For this review, use the dimensioned drawing (mm, ordinates from the lowest corner) and the shaded views. A direction names the side the tool comes from. Coordinates: 2 decimals unless noted, no trailing zeros. Order: outer loops, then holes, each group sorted by start corner. A loop starts at its lowest first (then second) coordinate and runs counter-clockwise, first axis right, second up. Notation, with made-up numbers: M 34.25,47 L 62.25,47 A19 cw 62.25,54 Z; hole C 22,34 d5. An arc over 180 degrees is marked long. Answer in a Markdown table with one row per item.
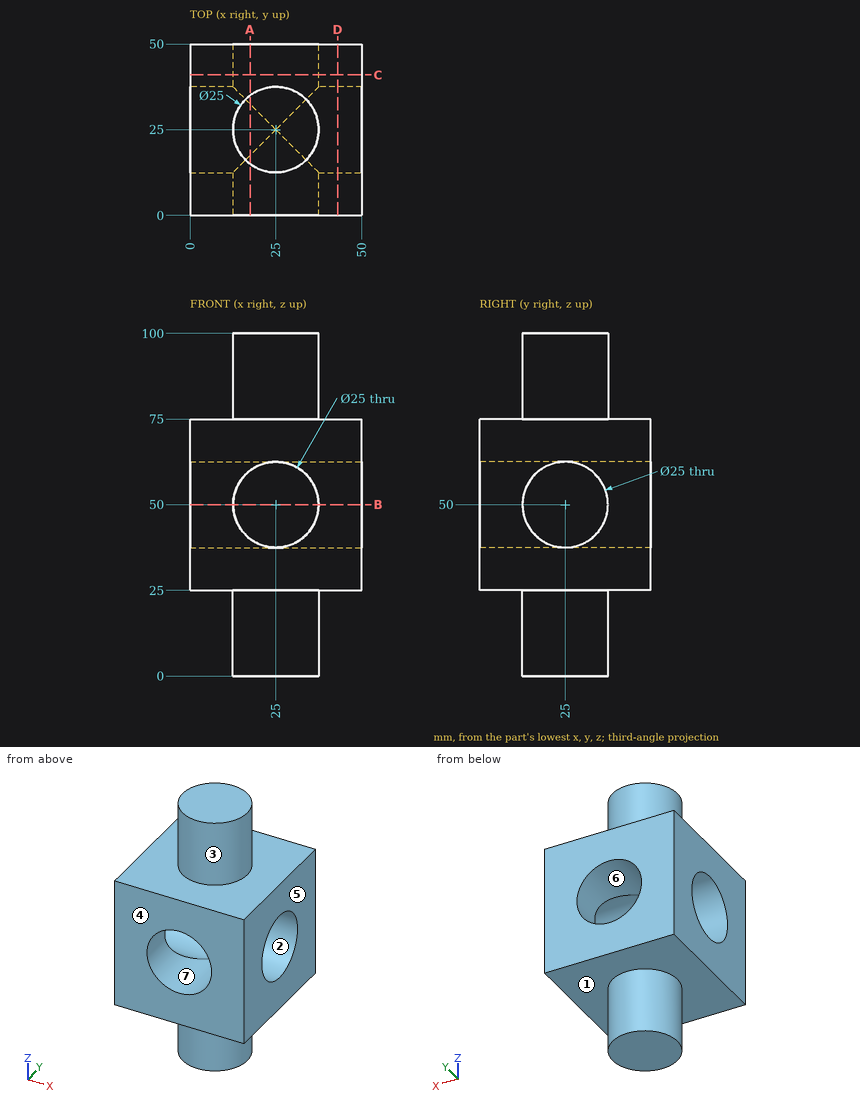
(1) Take a section at C-C (y = 41). Write out the cut boundary in (x, z), then the cut area to 3 significant figures.
Report:
| item | result |
|---|---|
| outline | M 0,25 L 50,25 L 50,75 L 0,75 Z; hole C 25,50 d25 |
| area | 2,010 mm^2 |
(2) Insertion check: P1, Ø8, axis at x = 10.5, y = 16, coming from the +Z side; P2, Ø15, axis at x = 25, z = 50, coming from the +Y side; P3, Ø6, axis at x = 35.5, z = 60.5, coming from the -Y side; P4, Ø2, axis at y = 12.5, z = 11.5, coming from the -X side. Each pin has a flat end and moves straight along its axis. Give the tip position at first contact, or say it passes through.
Report:
| item | result |
|---|---|
| P1 | z = 75 |
| P2 | through |
| P3 | y = 0 |
| P4 | x = 20.1 |
(3) To check wall thickness, follow line 1 (Z direction, x = 25, y = 18); line 2 (Y direction, x = 10.75, z = 50); line 3 (Z direction, x = 43, y = 25). State the ranges of each line that lie inside material, in increasing order. Write a range as [from, to].
Report:
| item | result |
|---|---|
| line 1 | [0, 37.5], [62.5, 100] |
| line 2 | [0, 12.5], [37.5, 50] |
| line 3 | [25, 37.5], [62.5, 75] |
(4) Take a section at B-B (z = 50). Write out the cut boundary in (x, y).
Report:
| item | result |
|---|---|
| outline | M 0,0 L 12.5,0 L 12.5,12.5 L 0,12.5 Z; M 0,37.5 L 12.5,37.5 L 12.5,50 L 0,50 Z; M 37.5,0 L 50,0 L 50,12.5 L 37.5,12.5 Z; M 37.5,37.5 L 50,37.5 L 50,50 L 37.5,50 Z |
(5) The part is to be moulded in two halves that separate along X. For the marked faces 4, 5, 6 and 7, say which applies: +X half, -X half, draft (parallel to the pull), parting line (faces both ways), or undercut.
Report:
| item | result |
|---|---|
| face 4 | draft |
| face 5 | +X half |
| face 6 | undercut |
| face 7 | undercut |
(6) Machinability: for the marked faces 1, 2 and 3, which of the approach directions +Z, -Z, +X, -X, +Y, -Y give a long, thin tool a straight path to every point of the face, cutting with its end or side? Answer none if there is none.
Report:
| item | result |
|---|---|
| face 1 | -Z |
| face 2 | +X, -X |
| face 3 | +Z |
(7) Take a section at A-A (x = 17.5). Write out the cut boundary in (y, z).
Report:
| item | result |
|---|---|
| outline | M 0,25 L 15,25 L 15,0 L 35,0 L 35,25 L 50,25 L 50,40 L 32.5,40 A12.5 cw 17.5,40 L 0,40 Z; M 0,60 L 17.5,60 A12.5 cw 32.5,60 L 50,60 L 50,75 L 35,75 L 35,100 L 15,100 L 15,75 L 0,75 Z |
